Design review of the part shown in the three views and the two pictorial views. Dimensions are in mm from the part's minimum x, y and z. A direction names the side the tool comes from. Round coordinates to 2 decimals unless told otherwise and drop trailing zeros. Order: outer loops, then holes, each group sorted by start corner. A loop starts at its lowest first (then second) coordinate and runs counter-clockwise, first axis right, second up.
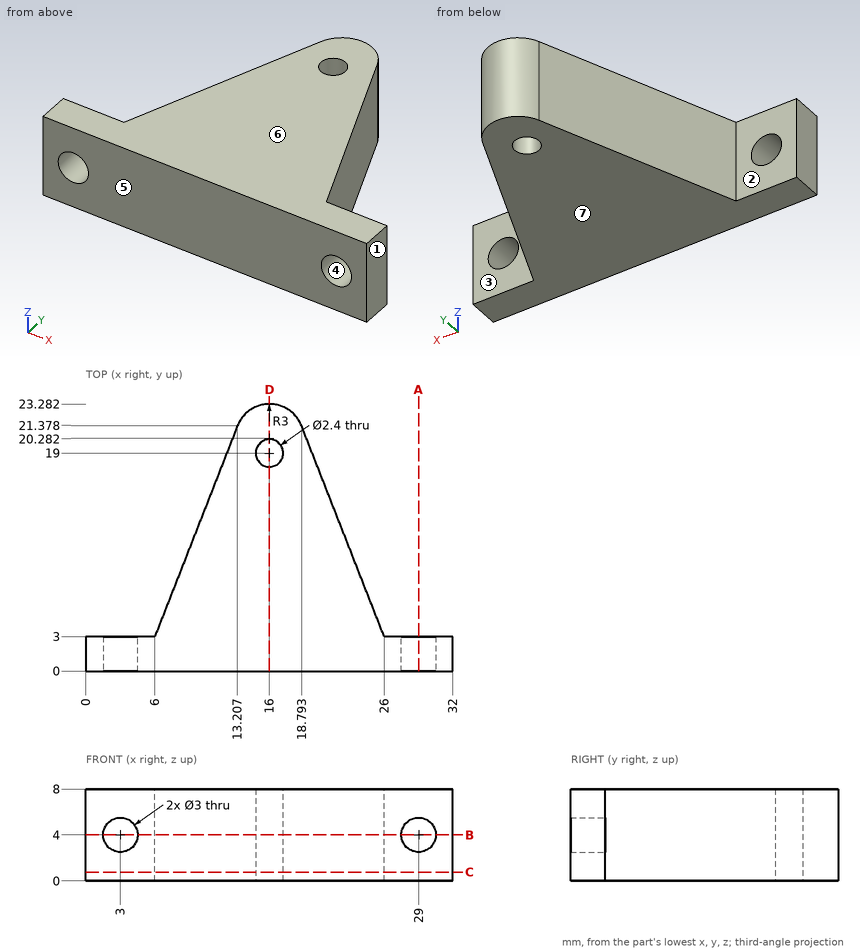
1) Take a section at C-C on z = 0.75. Give the boundary of the cut face in (x, y).
Results:
outline: (0, 0) - (32, 0) - (32, 3) - (26, 3) - (18.79, 21.38) arc R3 ccw to (13.21, 21.38) - (6, 3) - (0, 3) - close; hole circle Ø2.4 at (16, 19)
2) Take a section at B-B on z = 4. Give the boundary of the cut face in (x, y).
Results:
outline: (0, 0) - (1.5, 0) - (1.5, 3) - (0, 3) - close; (4.5, 0) - (27.5, 0) - (27.5, 3) - (26, 3) - (18.79, 21.38) arc R3 ccw to (13.21, 21.38) - (6, 3) - (4.5, 3) - close; (30.5, 0) - (32, 0) - (32, 3) - (30.5, 3) - close; hole circle Ø2.4 at (16, 19)
3) Take a section at D-D on x = 16. Give the boundary of the cut face in (y, z).
Results:
outline: (0, 0) - (17.8, 0) - (17.8, 8) - (0, 8) - close; (20.2, 0) - (23.28, 0) - (23.28, 8) - (20.2, 8) - close
4) The part is to be moulded in two halves that separate along Z. For the marked faces 4, 5, 6 and 7, say which applies: released by +Z, released by -Z, zero draft, split by the parting line, or undercut.
Results:
face 4: undercut
face 5: zero draft
face 6: released by +Z
face 7: released by -Z
5) Take a section at A-A on x = 29. Give the boundary of the cut face in (y, z), plus the area to 3 significant figures.
Results:
outline: (0, 0) - (3, 0) - (3, 2.5) - (0, 2.5) - close; (0, 5.5) - (3, 5.5) - (3, 8) - (0, 8) - close
area: 15.0 mm2
6) To check wall thickness, follow line 1 along Z through (x, y) = (29, 0.8); line 2 along Y through (x, z) = (27, 3); line 3 along Y through (x, z) = (16.5, 5). State the ranges of each line that lie inside material, in increasing order.
Results:
line 1: z = 0 to 2.5, 5.5 to 8
line 2: y = 0 to 3
line 3: y = 0 to 17.91, 20.09 to 23.24
7) For the marked faces 1, 2 and 3, list the 3-axis set-ups (+Z, -Z, +X, -X, +Y, -Y) from which the entire face can be reached by the end or side of a thin tool; tool diameter is ignored.
Results:
face 1: +Z, -Z, +X, +Y, -Y
face 2: +Z, -Z, -X, +Y
face 3: +Z, -Z, +X, +Y
8) Clearance check with flat-ended pins moving along their axes: P1, Ø1.5, axis at y = 8.5, z = 3.5, coming from the +X side; P2, Ø3.5, axis at x = 3, z = 4, coming from the +Y side. State where each tip first meets the part, or that it passes through.
Results:
P1: stops at x = 24.14
P2: stops at y = 3
